Geometry: final body of the model. Coordinates: model frame, mm. A direction names the side the tool comes from. Give positions to 0.01 mm unless a question says otherwise; leave off trailing zeros. Loops run counter-clockwise (first coordinate to the right, second up) from the corner with the lowest first, then second, coordinate; pieces in that order, holes last. Notation, with made-up numbers: (46.25, -3.75) - (102.25, -3.75) arc R9 ccw to (102.25, 9.25) - close; hole circle Ø7 at (-39.5, -19.5). An arc over 180 degrees is marked (long way). Use one line per item in the form item = value.
```python
from build123d import *

# Parameters (mm, degrees)
MODEL_W             = 101.6
MODEL_H             = 398.78
BOSS_EXTRUDE1_DEPTH = 6.35
SKETCH1_W           = 6.35
SKETCH1_H           = 10.16
CUT_EXTRUDE1_DEPTH  = 6.35
SKETCH2_W           = 95.776452478
SKETCH2_H           = 26.67
BOSS_EXTRUDE2_DEPTH = 6.35
SKETCH3_W           = 19.05
SKETCH3_H           = 6.35
SKETCH3_W_2         = 12.7
CUT_EXTRUDE2_DEPTH  = 6.35


with BuildPart() as part:
    # Model → Boss-Extrude1 (new body)
    with BuildSketch(Plane.XY):
        with Locations((50.8, 199.39)):
            Rectangle(MODEL_W, MODEL_H)
        with BuildLine():
            Line((77.47, 87.63), (20.83121403, 87.63))
            ThreePointArc((20.83121403, 87.63), (18.406749642, 85.847345646), (19.385420684, 83.001631833))
            Line((19.385420684, 83.001631833), (91.264206654, 33.239395393))
            ThreePointArc((91.264206654, 33.239395393), (93.888830968, 33.077884107), (95.25, 35.32776356))
            Line((95.25, 35.32776356), (95.25, 69.85))
            ThreePointArc((95.25, 69.85), (90.042358569, 82.422358569), (77.47, 87.63))
        make_face(mode=Mode.SUBTRACT)
        with BuildLine():
            Line((5.110654516, 145.400145775), (5.110654516, 110.877909335))
            ThreePointArc((5.110654516, 110.877909335), (6.471823548, 108.628029883), (9.096447862, 108.789541168))
            Line((9.096447862, 108.789541168), (80.975233831, 158.551777608))
            ThreePointArc((80.975233831, 158.551777608), (81.953904874, 161.397491422), (79.529440485, 163.180145775))
            Line((79.529440485, 163.180145775), (22.890654516, 163.180145775))
            ThreePointArc((22.890654516, 163.180145775), (10.318295946, 157.972504345), (5.110654516, 145.400145775))
        make_face(mode=Mode.SUBTRACT)
        with BuildLine():
            Line((77.47, 240.03), (20.83121403, 240.03))
            ThreePointArc((20.83121403, 240.03), (18.406749642, 238.247345646), (19.385420684, 235.401631833))
            Line((19.385420684, 235.401631833), (91.264206654, 185.639395393))
            ThreePointArc((91.264206654, 185.639395393), (93.888830968, 185.477884107), (95.25, 187.72776356))
            Line((95.25, 187.72776356), (95.25, 222.25))
            ThreePointArc((95.25, 222.25), (90.042358569, 234.822358569), (77.47, 240.03))
        make_face(mode=Mode.SUBTRACT)
        with BuildLine():
            Line((22.890654516, 175.880145775), (79.529440485, 175.880145775))
            ThreePointArc((79.529440485, 175.880145775), (81.953904874, 177.662800129), (80.975233831, 180.508513942))
            Line((80.975233831, 180.508513942), (9.096447862, 230.270750382))
            ThreePointArc((9.096447862, 230.270750382), (6.471823548, 230.432261668), (5.110654516, 228.182382216))
            Line((5.110654516, 228.182382216), (5.110654516, 193.660145775))
            ThreePointArc((5.110654516, 193.660145775), (10.318295946, 181.087787206), (22.890654516, 175.880145775))
        make_face(mode=Mode.SUBTRACT)
        with BuildLine():
            Line((91.264206654, 154.720604607), (19.385420684, 104.958368167))
            ThreePointArc((19.385420684, 104.958368167), (18.406749642, 102.112654354), (20.83121403, 100.33))
            Line((20.83121403, 100.33), (77.47, 100.33))
            ThreePointArc((77.47, 100.33), (90.042358569, 105.537641431), (95.25, 118.11))
            Line((95.25, 118.11), (95.25, 152.63223644))
            ThreePointArc((95.25, 152.63223644), (93.888830968, 154.882115893), (91.264206654, 154.720604607))
        make_face(mode=Mode.SUBTRACT)
        with BuildLine():
            Line((5.110654516, 297.800145775), (5.110654516, 263.277909335))
            ThreePointArc((5.110654516, 263.277909335), (6.471823548, 261.028029883), (9.096447862, 261.189541168))
            Line((9.096447862, 261.189541168), (80.975233831, 310.951777608))
            ThreePointArc((80.975233831, 310.951777608), (81.953904874, 313.797491422), (79.529440485, 315.580145775))
            Line((79.529440485, 315.580145775), (22.890654516, 315.580145775))
            ThreePointArc((22.890654516, 315.580145775), (10.318295946, 310.372504345), (5.110654516, 297.800145775))
        make_face(mode=Mode.SUBTRACT)
        with BuildLine():
            Line((88.9, 392.43), (20.83121403, 392.43))
            ThreePointArc((20.83121403, 392.43), (18.406749642, 390.647345646), (19.385420684, 387.801631833))
            Line((19.385420684, 387.801631833), (91.264206654, 338.039395393))
            ThreePointArc((91.264206654, 338.039395393), (93.888830968, 337.877884107), (95.25, 340.12776356))
            Line((95.25, 340.12776356), (95.25, 386.08))
            ThreePointArc((95.25, 386.08), (93.390128061, 390.570128061), (88.9, 392.43))
        make_face(mode=Mode.SUBTRACT)
        with BuildLine():
            Line((22.890654516, 328.280145775), (79.529440485, 328.280145775))
            ThreePointArc((79.529440485, 328.280145775), (81.953904874, 330.062800129), (80.975233831, 332.908513942))
            Line((80.975233831, 332.908513942), (9.096447862, 382.670750382))
            ThreePointArc((9.096447862, 382.670750382), (6.471823548, 382.832261668), (5.110654516, 380.582382216))
            Line((5.110654516, 380.582382216), (5.110654516, 346.060145775))
            ThreePointArc((5.110654516, 346.060145775), (10.318295946, 333.487787206), (22.890654516, 328.280145775))
        make_face(mode=Mode.SUBTRACT)
        with BuildLine():
            Line((22.890654516, 30.48), (85.626201641, 30.48))
            Line((85.626201641, 30.48), (10.005950978, 74.34818594))
            ThreePointArc((10.005950978, 74.34818594), (8.258764757, 77.658550083), (5.110654516, 75.633563082))
            Line((5.110654516, 75.633563082), (5.110654516, 48.26))
            ThreePointArc((5.110654516, 48.26), (10.318295946, 35.687641431), (22.890654516, 30.48))
        make_face(mode=Mode.SUBTRACT)
        with BuildLine():
            Line((91.264206654, 307.120604607), (19.385420684, 257.358368167))
            ThreePointArc((19.385420684, 257.358368167), (18.406749642, 254.512654354), (20.83121403, 252.73))
            Line((20.83121403, 252.73), (77.47, 252.73))
            ThreePointArc((77.47, 252.73), (90.042358569, 257.937641431), (95.25, 270.51))
            Line((95.25, 270.51), (95.25, 305.03223644))
            ThreePointArc((95.25, 305.03223644), (93.888830968, 307.282115893), (91.264206654, 307.120604607))
        make_face(mode=Mode.SUBTRACT)
    extrude(amount=BOSS_EXTRUDE1_DEPTH)

    # Sketch1 → Cut-Extrude1 (cut)
    with BuildSketch(Plane.XY.offset(6.35)):
        with Locations((98.425, 323.200145775)):
            Rectangle(SKETCH1_W, SKETCH1_H)
        with Locations((98.425, 247.65)):
            Rectangle(SKETCH1_W, SKETCH1_H)
        with Locations((3.175, 247.65)):
            Rectangle(SKETCH1_W, SKETCH1_H)
        with Locations((3.175, 25.4)):
            Rectangle(SKETCH1_W, SKETCH1_H)
        with Locations((98.425, 170.800145775)):
            Rectangle(SKETCH1_W, SKETCH1_H)
        with Locations((3.175, 323.200145775)):
            Rectangle(SKETCH1_W, SKETCH1_H)
        with Locations((98.425, 25.4)):
            Rectangle(SKETCH1_W, SKETCH1_H)
        with Locations((98.425, 95.25)):
            Rectangle(SKETCH1_W, SKETCH1_H)
        with Locations((3.175, 95.25)):
            Rectangle(SKETCH1_W, SKETCH1_H)
        with Locations((3.175, 170.800145775)):
            Rectangle(SKETCH1_W, SKETCH1_H)
    extrude(amount=-CUT_EXTRUDE1_DEPTH, mode=Mode.SUBTRACT)

    # Sketch2 → Boss-Extrude2 (add)
    with BuildSketch(Plane.XY.offset(6.35)):
        with Locations((49.666030554, 226.695)):
            Rectangle(SKETCH2_W, SKETCH2_H)
    extrude(amount=-BOSS_EXTRUDE2_DEPTH)

    # Sketch3 → Cut-Extrude2 (cut)
    with BuildSketch(Plane.XY.offset(6.35)):
        with Locations((79.375, 224.155)):
            Rectangle(SKETCH3_W, SKETCH3_H)
        with Locations((22.225, 224.155)):
            Rectangle(SKETCH3_W, SKETCH3_H)
        with Locations((50.8, 224.155)):
            Rectangle(SKETCH3_W_2, SKETCH3_H)
    extrude(amount=-CUT_EXTRUDE2_DEPTH, mode=Mode.SUBTRACT)


solid = part.part
```
(1) Cut plane A-A (y = 267). Return the cut outline in (x, z), plus the area to 3 significant figures.
Solution:
outline = (0, 0) - (5.11, 0) - (5.11, 6.35) - (0, 6.35) - close; (17.49, 0) - (33.31, 0) - (33.31, 6.35) - (17.49, 6.35) - close; (94.9, 0) - (101.6, 0) - (101.6, 6.35) - (94.9, 6.35) - close
area = 175 mm2
(2) Access query for faces 4 (the face through (101.6, 10, 3)), 5 (the face through (0, 10, 3)), 6 (the face through (52, 315.58, 3)), 7 (the face through (95.25, 171, 3)), 8 (the face through (6.35, 25, 3)). Directions: +Z, -Z, +X, -X, +Y, -Y. A direction counts if a zero-diameter tool reaches every point of the face in a straight line with its end or side. Return the directions, or none.
Solution:
face_4 = +Z, -Z, +X, +Y, -Y
face_5 = +Z, -Z, -X, +Y, -Y
face_6 = +Z, -Z
face_7 = +Z, -Z, +X
face_8 = +Z, -Z, -X
(3) Cut plane C-C (y = 52). Return the cut outline in (x, z).
Solution:
outline = (0, 0) - (5.11, 0) - (5.11, 6.35) - (0, 6.35) - close; (48.53, 0) - (64.17, 0) - (64.17, 6.35) - (48.53, 6.35) - close; (95.25, 0) - (101.6, 0) - (101.6, 6.35) - (95.25, 6.35) - close
(4) Pull-direction query (Y, two-part tool) for faces 1 (the face through (50.1, 202.2, 6.35)), 2 (the face through (98, 90.17, 3)), 3 (the face through (51, 175.88, 3)); classes: released by +Y, released by -Y, zero draft, split by the parting line, or undercut.
Solution:
face_1 = zero draft
face_2 = undercut
face_3 = undercut
(5) Pin query (flat end, axial travel): P1, Ø12, axis at x = 72.5, y = 223, coming from the -Z side; P2, Ø1.9, axis at y = 248.5, z = 3.5, coming from the +X side. Return the tip coordinate at first contact, or that it passes through.
Solution:
P1 = 0
P2 = 95.25
(6) Cut plane B-B (z = 2.25). Give the number of separate pieces and of enclosed holes in the cut face, plus the area to 3 significant figures.
Solution:
separate_pieces = 1
enclosed_holes = 13
area = 19,100 mm2
(7) Material intervals for L1, parallel to Y at x = 9.5, z = 1.75; L2, parallel to X at y = 66, z = 2.75; L3, parallel to X at y = 212.5, z = 4, sorted ascending. Write a range as from..to.
Solution:
L1 = 0..36.56, 76.9..109.07, 157.1..181.96, 213.36..261.47, 309.5..334.36, 382.39..398.78
L2 = 0..5.11, 24.4..43.94, 95.25..101.6
L3 = 0..5.11, 34.77..52.47, 95.25..101.6
